Geometry check sheet. Reference: the model listing, model coordinates, mm. A direction names the side the tool comes from. Coordinates: 2 decimals unless noted, no trailing zeros. Write each loop counter-clockwise with the first axis right and the second up, starting at its lowest first coordinate (ties: lowest second). Pieces come first, ordered by that corner, then holes. Notation, with made-up numbers: M -4.5,69 L 13.5,69 A18 ccw 13.5,77 Z; hole C 75.5,-3.75 d10. An arc over 180 degrees is marked long. Write each question's results on one line, items separated by ' | '.
```python
from build123d import *

# Parameters (mm, degrees)
F0_W     = 66.549368
F0_H     = 4.092034
F0_H_2   = 4.307404
F1_DEPTH = 25.4
F2_DEPTH = 50.8
F3_R     = 8.033842
F4_DEPTH = 131.064


with BuildPart() as f1:
    # F0 (on Top) → F1 (new body)
    with BuildSketch(Plane.XY):
        with Locations((-0.21537, -31.337576)):
            Rectangle(F0_W, F0_H)
        Polygon((-62.780388, 30.150594), (-62.780388, -33.383593), (-33.490054, -33.383593), (-33.490054, -29.291559), (-58.472987, -29.291559), (-58.472987, 25.84319), (-33.490054, 25.84319), (-33.490054, 30.150594), align=None)
        with Locations((-0.21537, 27.996892)):
            Rectangle(F0_W, F0_H_2)
        Polygon((33.059314, -29.291559), (33.059314, -33.383593), (66.657059, -33.383593), (66.657059, 30.150594), (33.059314, 30.150594), (33.059314, 25.84319), (62.134281, 25.84319), (62.134281, -29.291559), align=None)
    extrude(amount=F1_DEPTH)

    # F0 (on Top) → F2 (join)
    with BuildSketch(Plane.XY):
        Polygon((-62.780388, 30.150594), (-62.780388, -33.383593), (-33.490054, -33.383593), (-33.490054, -29.291559), (-58.472987, -29.291559), (-58.472987, 25.84319), (-33.490054, 25.84319), (-33.490054, 30.150594), align=None)
        Polygon((33.059314, -29.291559), (33.059314, -33.383593), (66.657059, -33.383593), (66.657059, 30.150594), (33.059314, 30.150594), (33.059314, 25.84319), (62.134281, 25.84319), (62.134281, -29.291559), align=None)
    extrude(amount=F2_DEPTH)

    # F3 (on face) → F4 (cut)
    with BuildSketch(Plane.YZ.offset(66.657059)):
        with Locations((0, 22.118356)):
            Circle(F3_R)
    extrude(amount=-F4_DEPTH, mode=Mode.SUBTRACT)


solid = f1.part
```
Q1. Sectioned sample at D-D on y = -14.5. Record the cut outline in (x, z).
Geometry check:
outline: M -62.78,0 L -58.47,0 L -58.47,50.8 L -62.78,50.8 Z; M 62.13,0 L 66.66,0 L 66.66,50.8 L 62.13,50.8 Z
Q2. Access from +Z, -Z, +X, -X, +Y, -Y to the whole of each face (thin tool, end or side, straight path). Record for faces 1 (the flat face through (-58.473, -2, 31)), 2 (the flat face through (-33.49, 28, 38)), 3 (the flat face through (-62.78, -1, 31)).
Geometry check:
face 1: +Z, -Z | face 2: +Z, +Y, -Y | face 3: +Z, -Z, -X, +Y, -Y
Q3. Sectioned sample at A-A on x = 49. Record the cut outline in (y, z), and give its area (3 significant figures).
Geometry check:
outline: M -33.38,0 L -29.29,0 L -29.29,50.8 L -33.38,50.8 Z; M 25.84,0 L 30.15,0 L 30.15,50.8 L 25.84,50.8 Z | area: 427 mm2
Q4. Depth check by flat-ended pin: P1, Ø1.3, axis at x = -7.5, y = 28.5, coming from the +Z side; P2, Ø18.5, axis at y = 0, z = 22.12, coming from the -X side. Enter the tip coordinate at first touch or a pass-through.
Geometry check:
P1: stops at z = 25.4 | P2: stops at x = -62.78
Q5. Sectioned sample at C-C on y = 0. Record the cut outline in (x, z), and give its area (3 significant figures).
Geometry check:
outline: M -62.78,0 L -58.47,0 L -58.47,14.08 L -62.78,14.08 Z; M -62.78,30.15 L -58.47,30.15 L -58.47,50.8 L -62.78,50.8 Z; M 62.13,0 L 66.66,0 L 66.66,14.08 L 62.13,14.08 Z; M 62.13,30.15 L 66.66,30.15 L 66.66,50.8 L 62.13,50.8 Z | area: 307 mm2
Q6. Mould release check, pull along Z, two halves, no side actions. Record for faces 4 (the flat face through (-59, -4, 50.8)), 5 (the flat face through (1, 25.843, 19)), 6 (the cylindrical face through (-60.597, -1.046, 30.084)): pulls with the +Z half, pulls with the -Z half, needs draft (parallel to the pull), parting line crosses it, or undercut.
Geometry check:
face 4: pulls with the +Z half | face 5: needs draft | face 6: undercut
Q7. Scan lines: probe 1 along X at (y, z) = (18.5, 37.5); probe 2 along Y at (x, z) = (45, 16); probe 3 along Z at (x, y) = (-61, 0). Record each from-to range of solid material in increasing order.
Geometry check:
probe 1: x = -62.78 to -58.47, 62.13 to 66.66 | probe 2: y = -33.38 to -29.29, 25.84 to 30.15 | probe 3: z = 0 to 14.08, 30.15 to 50.8
Q8. Sectioned sample at B-B on z = 6.5. Record the cut outline in (x, y), and give its area (3 significant figures).
Geometry check:
outline: M -62.78,-33.38 L 66.66,-33.38 L 66.66,30.15 L -62.78,30.15 Z; hole M -58.47,-29.29 L 62.13,-29.29 L 62.13,25.84 L -58.47,25.84 Z | area: 1,570 mm2
